from build123d import *

# Parameters (mm, degrees)
SKETCH1_R           = 71.85
SKETCH1_R_2         = 56.85
BOSS_EXTRUDE1_DEPTH = 5
CUT_EXTRUDE1_DEPTH  = 2
CUT_EXTRUDE2_REACH  = 103.734
SKETCH3_R           = 1.6


with BuildPart() as part:
    # Sketch1 → Boss-Extrude1 (new body)
    with BuildSketch(Plane(origin=(0, 0, 0), x_dir=(0, 0, -1), z_dir=(1, 0, 0))):
        Circle(SKETCH1_R)
        Circle(SKETCH1_R_2, mode=Mode.SUBTRACT)
    extrude(amount=BOSS_EXTRUDE1_DEPTH)

    # Sketch2 → Cut-Extrude1 (cut)
    with BuildSketch(Plane(origin=(5, 0, 0), x_dir=(0, 0, -1), z_dir=(1, 0, 0))):
        Polygon((54.790689352, 31.633419246), (57.590689352, 30.016838493), (60.390689352, 31.633419246), (60.390689352, 34.866580754), (57.590689352, 36.483161507), (54.790689352, 34.866580754), align=None)
        Polygon((0, 63.266838493), (2.8, 64.883419246), (2.8, 68.116580754), (0, 69.733161507), (-2.8, 68.116580754), (-2.8, 64.883419246), align=None)
        Polygon((54.790689352, -31.633419246), (54.790689352, -34.866580754), (57.590689352, -36.483161507), (60.390689352, -34.866580754), (60.390689352, -31.633419246), (57.590689352, -30.016838493), align=None)
        Polygon((0, -63.266838493), (-2.8, -64.883419246), (-2.8, -68.116580754), (0, -69.733161507), (2.8, -68.116580754), (2.8, -64.883419246), align=None)
        Polygon((-54.790689352, -31.633419246), (-57.590689352, -30.016838493), (-60.390689352, -31.633419246), (-60.390689352, -34.866580754), (-57.590689352, -36.483161507), (-54.790689352, -34.866580754), align=None)
        Polygon((-54.790689352, 31.633419246), (-54.790689352, 34.866580754), (-57.590689352, 36.483161507), (-60.390689352, 34.866580754), (-60.390689352, 31.633419246), (-57.590689352, 30.016838493), align=None)
    extrude(amount=-CUT_EXTRUDE1_DEPTH, mode=Mode.SUBTRACT)

    # Sketch3 → Cut-Extrude2 (cut, up to next)
    with BuildSketch(Plane(origin=(5, 0, 0), x_dir=(0, 0, -1), z_dir=(1, 0, 0)), mode=Mode.PRIVATE) as cut_extrude2_sk1:
        with Locations((0, 66.5)):
            Circle(SKETCH3_R)
    cut_extrude2_tool1 = extrude(cut_extrude2_sk1.sketch, amount=-CUT_EXTRUDE2_REACH, mode=Mode.PRIVATE) & part.part
    # Sketch3 → Cut-Extrude2 (cut, up to next)
    with BuildSketch(Plane(origin=(5, 0, 0), x_dir=(0, 0, -1), z_dir=(1, 0, 0)), mode=Mode.PRIVATE) as cut_extrude2_sk2:
        with Locations((57.590689352, 33.25)):
            Circle(SKETCH3_R)
    cut_extrude2_tool2 = extrude(cut_extrude2_sk2.sketch, amount=-CUT_EXTRUDE2_REACH, mode=Mode.PRIVATE) & part.part
    # Sketch3 → Cut-Extrude2 (cut, up to next)
    with BuildSketch(Plane(origin=(5, 0, 0), x_dir=(0, 0, -1), z_dir=(1, 0, 0)), mode=Mode.PRIVATE) as cut_extrude2_sk3:
        with Locations((57.590689352, -33.25)):
            Circle(SKETCH3_R)
    cut_extrude2_tool3 = extrude(cut_extrude2_sk3.sketch, amount=-CUT_EXTRUDE2_REACH, mode=Mode.PRIVATE) & part.part
    # Sketch3 → Cut-Extrude2 (cut, up to next)
    with BuildSketch(Plane(origin=(5, 0, 0), x_dir=(0, 0, -1), z_dir=(1, 0, 0)), mode=Mode.PRIVATE) as cut_extrude2_sk4:
        with Locations((0, -66.5)):
            Circle(SKETCH3_R)
    cut_extrude2_tool4 = extrude(cut_extrude2_sk4.sketch, amount=-CUT_EXTRUDE2_REACH, mode=Mode.PRIVATE) & part.part
    # Sketch3 → Cut-Extrude2 (cut, up to next)
    with BuildSketch(Plane(origin=(5, 0, 0), x_dir=(0, 0, -1), z_dir=(1, 0, 0)), mode=Mode.PRIVATE) as cut_extrude2_sk5:
        with Locations((-57.590689352, -33.25)):
            Circle(SKETCH3_R)
    cut_extrude2_tool5 = extrude(cut_extrude2_sk5.sketch, amount=-CUT_EXTRUDE2_REACH, mode=Mode.PRIVATE) & part.part
    # Sketch3 → Cut-Extrude2 (cut, up to next)
    with BuildSketch(Plane(origin=(5, 0, 0), x_dir=(0, 0, -1), z_dir=(1, 0, 0)), mode=Mode.PRIVATE) as cut_extrude2_sk6:
        with Locations((-57.590689352, 33.25)):
            Circle(SKETCH3_R)
    cut_extrude2_tool6 = extrude(cut_extrude2_sk6.sketch, amount=-CUT_EXTRUDE2_REACH, mode=Mode.PRIVATE) & part.part
    add(cut_extrude2_tool1.solids().sort_by_distance((5, 66.5, 0))[0], mode=Mode.SUBTRACT)
    add(cut_extrude2_tool2.solids().sort_by_distance((5, 33.25, -57.590689))[0], mode=Mode.SUBTRACT)
    add(cut_extrude2_tool3.solids().sort_by_distance((5, -33.25, -57.590689))[0], mode=Mode.SUBTRACT)
    add(cut_extrude2_tool4.solids().sort_by_distance((5, -66.5, 0))[0], mode=Mode.SUBTRACT)
    add(cut_extrude2_tool5.solids().sort_by_distance((5, -33.25, 57.590689))[0], mode=Mode.SUBTRACT)
    add(cut_extrude2_tool6.solids().sort_by_distance((5, 33.25, 57.590689))[0], mode=Mode.SUBTRACT)

    # Sketch4 → Cut-Revolve1 (revolve, cut)
    with BuildSketch(Plane.XY, mode=Mode.PRIVATE) as cut_revolve1_sk:
        Polygon((0, -71.35), (0, -71.85), (5, -71.85), align=None)
    revolve(cut_revolve1_sk.sketch.rotate(Axis((0, 0, 0), (1, 0, 0)), 270), axis=Axis((0, 0, 0), (1, 0, 0)), mode=Mode.SUBTRACT)


solid = part.part
Here's how the part is built. I have some questions about the finished solid (model axes, mm). A direction names the side the tool comes from. Coordinates: 2 decimals unless noted, no trailing zeros. Order: outer loops, then holes, each group sorted by start corner. A loop starts at its lowest first (then second) coordinate and runs counter-clockwise, first axis right, second up. Notation, with made-up numbers: M 4.25,10 L 58.25,10 A28 ccw 58.25,32 Z; hole C 20.25,-19 d4. An arc over 180 degrees is marked long. Answer as CSV lines item,"result".
Item 1: On a 3-axis mill with a long thin cutter (end or side, diameter ignored), from which of +Z, -Z, +X, -X, +Y, -Y can I reach the whole of each face in a straight line? I mean faces 5 (the face through (3, -35, 59)), 6 (the face through (1.521, -64.914, 0.208)). Say none if no direction works.
Results found:
face 5,"+X"
face 6,"+X, -X"
Item 2: Imagine slicing it at B-B on x = 1.3. Write out the boundary of the cut face in (y, z), plus the area to 3 significant figures.
Results found:
outline,"C 0,0 d142.96; hole C -66.5,0 d3.2; hole C 0,0 d113.7; hole C -33.25,-57.59 d3.2; hole C -33.25,57.59 d3.2; hole C 33.25,-57.59 d3.2; hole C 33.25,57.59 d3.2; hole C 66.5,0 d3.2"
area,"5,850 mm2"
Item 3: We'd pull the mould along Y, two halves only. Please class faces 1 (the face through (1.52, -33.86, -59.07)), 2 (the face through (0.243, -21.439, 68.078)), 3 (the face through (0, -31, 48)), 4 (the face through (3, 65, 1)): +Y half, -Y half, draft (parallel to the pull), parting line (faces both ways), or undercut.
Results found:
face 1,"undercut"
face 2,"parting line"
face 3,"draft"
face 4,"undercut"
Item 4: If I drill on line 1 (Y direction, x = 2.3, z = 0); line 2 (Y direction, x = 4.45, z = 0) (3 decimals); line 3 (Z direction, x = 1.65, y = 35.5), over which ranges is the centre line in solid material (lowest first)?
Results found:
line 1,"-71.58 to -68.1, -64.9 to -56.85, 56.85 to 64.9, 68.1 to 71.58"
line 2,"-71.795 to -69.733, -63.267 to -56.85, 56.85 to 63.267, 69.733 to 71.795"
line 3,"-62.08 to -44.4, 44.4 to 62.08"
Item 5: For pin 1 (1 mm diameter, centred on x = 3.5, y = 33.5, fed in from -Z); pin 2 (1 mm diameter, centred on x = 3.5, y = 66, fed in from -Z); pin 3 (5 mm diameter, centred on y = 33.25, z = 57.59, fed in from +X); pin 4 (3 mm diameter, centred on y = 66.5, z = 0, fed in from +X), each with a flat end and sliding along its axis, tell me the tip position at first contact or that it passes through.
Results found:
pin 1,"z = -63.66"
pin 2,"z = -29.17"
pin 3,"x = 3"
pin 4,"through"
Item 6: Imagine slicing it at A-A on y = 0. Write out the boundary of the cut face in (x, z).
Results found:
outline,"M 0,-71.35 L 5,-71.85 L 5,-56.85 L 0,-56.85 Z; M 0,56.85 L 5,56.85 L 5,71.85 L 0,71.35 Z"
